```python
from build123d import *

# Parameters (mm, degrees)
BOSS_EXTRUDE1_DEPTH = 80.4
SKETCH2_R           = 3.175
CUT_EXTRUDE1_DEPTH  = 4.175
SKETCH3_R           = 1.5
SKETCH3_R_2         = 3
CUT_EXTRUDE2_DEPTH  = 39.1


with BuildPart() as part:
    # Sketch1 → Boss-Extrude1 (new body)
    with BuildSketch(Plane.XY):
        Polygon((0, 0), (3.175, 0), (3.175, 34.925), (45.475, 34.925), (45.475, 38.1), (0, 38.1), align=None)
    extrude(amount=BOSS_EXTRUDE1_DEPTH)

    # Sketch2 → Cut-Extrude1 (cut, through all)
    with BuildSketch(Plane(origin=(3.175, 0, 0), x_dir=(0, 0, -1), z_dir=(1, 0, 0))):
        with Locations((-70.875, 12.7)):
            Circle(SKETCH2_R)
        with Locations((-9.525, 12.7)):
            Circle(SKETCH2_R)
    extrude(amount=-CUT_EXTRUDE1_DEPTH, mode=Mode.SUBTRACT)

    # Sketch3 → Cut-Extrude2 (cut, through all)
    with BuildSketch(Plane(origin=(0, 38.1, 0), x_dir=(1, 0, 0), z_dir=(0, 1, 0))):
        with Locations((39.825, -55.7)):
            Circle(SKETCH3_R)
        with Locations((8.825, -55.7)):
            Circle(SKETCH3_R)
        with Locations((8.825, -24.7)):
            Circle(SKETCH3_R)
        with Locations((39.825, -24.7)):
            Circle(SKETCH3_R)
        with Locations((24.325, -40.2)):
            Circle(SKETCH3_R_2)
    extrude(amount=-CUT_EXTRUDE2_DEPTH, mode=Mode.SUBTRACT)


solid = part.part
```
Verification items for the finished model (mm, model axes). A direction names the side the tool comes from. Coordinates: 2 decimals unless noted, no trailing zeros. Order: outer loops, then holes, each group sorted by start corner. A loop starts at its lowest first (then second) coordinate and runs counter-clockwise, first axis right, second up. Notation, with made-up numbers: (45, -20.75) -> (55, -20.75) arc R19 cw to (55, -13.75) -> close; hole circle Ø2 at (36, -30). An arc over 180 degrees is marked (long way). Put each result on its own line as item: value. Start each with the question number.
1) Cross-section at D-D (x = 40.5). Enter the section's corners in (y, z) (3 decimals), plus the area to 3 significant figures.
2) Cross-section at B-B (y = 12.7). Enter the section's corners in (x, z) (3 decimals), plus the area to 3 significant figures.
3) Release check for a two-part mould opening along X. For faces 3 (the cylindrical face through (39.5, 36.535, 57.164)), 4 (the flat face through (0, 19, 40)), 5 (the cylindrical face through (1.61, 13.654, 67.847)), 6 (the flat face through (3.175, 17, 40)) record: pulls with the +X half, pulls with the -X half, needs draft (parallel to the pull), parting line crosses it, or undercut.
4) Cross-section at C-C (z = 40.2). Enter the section's corners in (x, y) (3 decimals), plus the area to 3 significant figures.
5) Go/stop test with flat-tipped pins: pin 1 (12 mm diameter, centred on y = 7.5, z = 45.5, fed in from +X) (3 decimals); pin 2 (3.5 mm diameter, centred on x = 8.825, z = 24.7, fed in from -Y) (3 decimals). Record where each tip stops, or that it passes through.
6) Material ranges on L1, parallel to X at y = 36.3, z = 55.7 (3 decimals); L2, parallel to X at y = 36.65, z = 40.2 (3 decimals); L3, parallel to Z at x = 2, y = 12, recorded low to high.
7) Tool access check on faces 1 (the flat face through (19, 34.925, 40)), 2 (the cylindrical face through (23.934, 36.535, 37.226)). Record the directions out of +Z, -Z, +X, -X, +Y, -Y that give a thin tool (end or side, any length) a straight path to the whole face; none if there is none.
8) Cross-section at A-A (z = 55.7). Enter the section's corners in (x, y) (3 decimals), plus the area to 3 significant figures.
Geometry check:
1. outline: (34.925, 0) -> (38.1, 0) -> (38.1, 23.36) -> (34.925, 23.36) -> close; (34.925, 26.04) -> (38.1, 26.04) -> (38.1, 54.36) -> (34.925, 54.36) -> close; (34.925, 57.04) -> (38.1, 57.04) -> (38.1, 80.4) -> (34.925, 80.4) -> close
1. area: 238 mm^2
2. outline: (0, 0) -> (3.175, 0) -> (3.175, 6.35) -> (0, 6.35) -> close; (0, 12.7) -> (3.175, 12.7) -> (3.175, 67.7) -> (0, 67.7) -> close; (0, 74.05) -> (3.175, 74.05) -> (3.175, 80.4) -> (0, 80.4) -> close
2. area: 215 mm^2
3. face 3: undercut
3. face 4: pulls with the -X half
3. face 5: needs draft
3. face 6: pulls with the +X half
4. outline: (0, 0) -> (3.175, 0) -> (3.175, 34.925) -> (21.325, 34.925) -> (21.325, 38.1) -> (0, 38.1) -> close; (27.325, 34.925) -> (45.475, 34.925) -> (45.475, 38.1) -> (27.325, 38.1) -> close
4. area: 236 mm^2
5. pin 1: stops at x = 3.175
5. pin 2: stops at y = 34.925
6. L1: x = 0 to 7.325, 10.325 to 38.325, 41.325 to 45.475
6. L2: x = 0 to 21.325, 27.325 to 45.475
6. L3: z = 0 to 6.43, 12.62 to 67.78, 73.97 to 80.4
7. face 1: +Z, -Z, +X, -Y
7. face 2: +Y, -Y
8. outline: (0, 0) -> (3.175, 0) -> (3.175, 34.925) -> (7.325, 34.925) -> (7.325, 38.1) -> (0, 38.1) -> close; (10.325, 34.925) -> (38.325, 34.925) -> (38.325, 38.1) -> (10.325, 38.1) -> close; (41.325, 34.925) -> (45.475, 34.925) -> (45.475, 38.1) -> (41.325, 38.1) -> close
8. area: 236 mm^2
